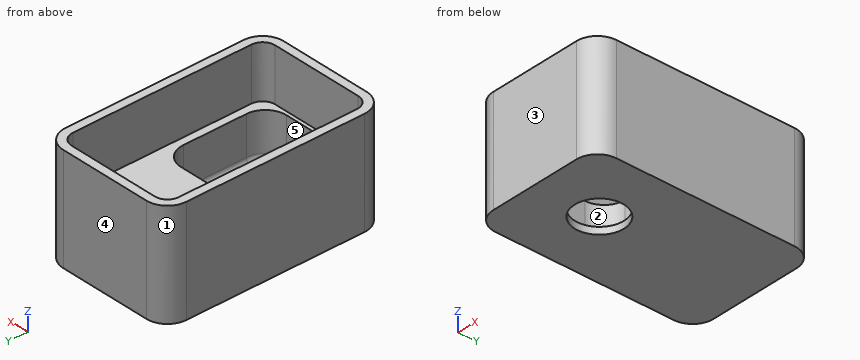
from build123d import *

# Parameters (mm, degrees)
SKETCH1_W           = 38.3
SKETCH1_H           = 62.8
SKETCH1_W_2         = 33.5
SKETCH1_H_2         = 58
SKETCH1_W_3         = 29
SKETCH1_H_3         = 30
SKETCH1_R           = 7
BOSS_EXTRUDE1_DEPTH = 2
BOSS_EXTRUDE2_START = 2
SKETCH1_3_W         = 38.3
SKETCH1_3_H         = 62.8
SKETCH1_3_W_2       = 33.5
SKETCH1_3_H_2       = 58
SKETCH1_3_W_3       = 29
SKETCH1_3_H_3       = 30
BOSS_EXTRUDE2_DEPTH = 13
BOSS_EXTRUDE3_START = 15
SKETCH1_4_W         = 38.3
SKETCH1_4_H         = 62.8
SKETCH1_4_W_2       = 33.5
SKETCH1_4_H_2       = 58
BOSS_EXTRUDE3_DEPTH = 15
FILLET1_R           = 3.6
FILLET2_R           = 6
FILLET3_R           = 2


with BuildPart() as part:
    # Sketch1 → Boss-Extrude1 (new body)
    # profile 1 of 3: a face of its own
    with BuildSketch(Plane.XY):
        with Locations((0, 13)):
            Rectangle(SKETCH1_W, SKETCH1_H)
        with Locations((0, 13)):
            Rectangle(SKETCH1_W_2, SKETCH1_H_2, mode=Mode.SUBTRACT)
    # profile 2 of 3: a face of its own
    with BuildSketch(Plane.XY):
        with Locations((0, 13)):
            Rectangle(SKETCH1_W_2, SKETCH1_H_2)
        Rectangle(SKETCH1_W_3, SKETCH1_H_3, mode=Mode.SUBTRACT)
    # profile 3 of 3: a face of its own
    with BuildSketch(Plane.XY):
        Rectangle(SKETCH1_W_3, SKETCH1_H_3)
        Circle(SKETCH1_R, mode=Mode.SUBTRACT)
    extrude(amount=BOSS_EXTRUDE1_DEPTH)

    # Sketch1<3> → Boss-Extrude2 (add)
    # profile 1 of 2: a face of its own
    with BuildSketch(Plane.XY.offset(BOSS_EXTRUDE2_START)):
        with Locations((0, 13)):
            Rectangle(SKETCH1_3_W, SKETCH1_3_H)
        with Locations((0, 13)):
            Rectangle(SKETCH1_3_W_2, SKETCH1_3_H_2, mode=Mode.SUBTRACT)
    # profile 2 of 2: a face of its own
    with BuildSketch(Plane.XY.offset(BOSS_EXTRUDE2_START)):
        with Locations((0, 13)):
            Rectangle(SKETCH1_3_W_2, SKETCH1_3_H_2)
        Rectangle(SKETCH1_3_W_3, SKETCH1_3_H_3, mode=Mode.SUBTRACT)
    extrude(amount=BOSS_EXTRUDE2_DEPTH)

    # Sketch1<4> → Boss-Extrude3 (add)
    with BuildSketch(Plane.XY.offset(BOSS_EXTRUDE3_START)):
        with Locations((0, 13)):
            Rectangle(SKETCH1_4_W, SKETCH1_4_H)
        with Locations((0, 13)):
            Rectangle(SKETCH1_4_W_2, SKETCH1_4_H_2, mode=Mode.SUBTRACT)
    extrude(amount=BOSS_EXTRUDE3_DEPTH)

    # Fillet1
    fillet1_edges = [part.edges().sort_by_distance(p)[0] for p in [
        (-16.75, 42, 22.5),
        (-16.75, -16, 22.5),
        (16.75, -16, 22.5),
        (16.75, 42, 22.5),
    ]]
    fillet(fillet1_edges, radius=FILLET1_R)

    # Fillet2
    fillet2_edges = [part.edges().sort_by_distance(p)[0] for p in [
        (19.15, -18.4, 15),
        (-19.15, -18.4, 15),
        (-19.15, 44.4, 15),
        (19.15, 44.4, 15),
        (14.5, -15, 8.5),
        (14.5, 15, 8.5),
        (-14.5, 15, 8.5),
        (-14.5, -15, 8.5),
    ]]
    fillet(fillet2_edges, radius=FILLET2_R)

    # Fillet3
    fillet3_edges = [part.edges().sort_by_distance(p)[0] for p in [
        (-14.5, 0, 2),
        (0, -15, 2),
        (14.5, 0, 2),
        (0, 15, 2),
        (12.742640687, 13.242640687, 2),
        (12.742640687, -13.242640687, 2),
        (-12.742640687, 13.242640687, 2),
        (-12.742640687, -13.242640687, 2),
    ]]
    fillet(fillet3_edges, radius=FILLET3_R)


solid = part.part
Can you work these out from the model? Positions are in its coordinate system, mm. Face numbers are marked on the shaded views. A direction names the side the tool comes from. Give positions to 0.01 mm unless a question says otherwise; leave off trailing zeros. Loops run counter-clockwise (first coordinate to the right, second up) from the corner with the lowest first, then second, coordinate; pieces in that order, holes last. Notation, with made-up numbers: (48.25, 88.25) - (68.25, 88.25) arc R28 cw to (68.25, 119.25) - close; hole circle Ø8 at (52.25, -20.5). An arc over 180 degrees is marked (long way). One line per item, written item: value.
(1) If we section it at C-C, the plane z = 8.5: List the corners of the cut face in (x, y) for me.
Verdict:
outline: (-19.15, -12.4) arc R6 ccw to (-13.15, -18.4) - (13.15, -18.4) arc R6 ccw to (19.15, -12.4) - (19.15, 38.4) arc R6 ccw to (13.15, 44.4) - (-13.15, 44.4) arc R6 ccw to (-19.15, 38.4) - close; hole (-14.5, -9) arc R6 ccw to (-8.5, -15) - (8.5, -15) arc R6 ccw to (14.5, -9) - (14.5, 9) arc R6 ccw to (8.5, 15) - (-8.5, 15) arc R6 ccw to (-14.5, 9) - close
(2) If we section it at B-B, the plane x = 0: List the corners of the cut face in (y, z) for me.
Verdict:
outline: (-18.4, 0) - (-7, 0) - (-7, 2) - (-13, 2) arc R2 cw to (-15, 4) - (-15, 15) - (-16, 15) - (-16, 30) - (-18.4, 30) - close; (7, 0) - (44.4, 0) - (44.4, 30) - (42, 30) - (42, 15) - (15, 15) - (15, 4) arc R2 cw to (13, 2) - (7, 2) - close
(3) If we section it at A-A, the plane y = 0: List the corners of the cut face in (x, z) for me, plus the area to 3 significant figures.
Verdict:
outline: (-19.15, 0) - (-7, 0) - (-7, 2) - (-12.5, 2) arc R2 cw to (-14.5, 4) - (-14.5, 15) - (-16.75, 15) - (-16.75, 30) - (-19.15, 30) - close; (7, 0) - (19.15, 0) - (19.15, 30) - (16.75, 30) - (16.75, 15) - (14.5, 15) - (14.5, 4) arc R2 cw to (12.5, 2) - (7, 2) - close
area: 243 mm^2
(4) I need wall thicknesses on line 1 along X through (y, z) = (-10, 27.75); line 2 along X through (y, z) = (8, 11.75); line 3 along Y through (x, z) = (0, 1.05). Which ranges of each line are inside material? Lowest first, please.
Verdict:
line 1: -19.15 to -16.75, 16.75 to 19.15
line 2: -19.15 to -14.5, 14.5 to 19.15
line 3: -18.4 to -7, 7 to 44.4
(5) I'm going to push flat-ended pins straight in: pin 1 (1 mm diameter, centred on x = 4, y = -3.5, fed in from +Z); pin 2 (3 mm diameter, centred on x = 8.5, y = 12, fed in from -Z); pin 3 (12.5 mm diameter, centred on x = -2, y = 5.5, fed in from +Z). Where does each tip first touch, or does it pass through?
Verdict:
pin 1: through
pin 2: z = 0
pin 3: z = 2
(6) If we section it at D-D, the plane y = 29: List the corners of the cut face in (x, z) for me.
Verdict:
outline: (-19.15, 0) - (19.15, 0) - (19.15, 30) - (16.75, 30) - (16.75, 15) - (-16.75, 15) - (-16.75, 30) - (-19.15, 30) - close
(7) If we mould it in two halves opening along X, with no side actions, what happens to the marked faces 1, 2 and 3? For each: released by +X, released by -X, zero draft, split by the parting line, or undercut.
Verdict:
face 1: released by -X
face 2: undercut
face 3: zero draft
(8) On a 3-axis mill with a long thin cutter (end or side, diameter ignored), from which of +Z, -Z, +X, -X, +Y, -Y can I reach the whole of each face in a straight line? I mean the marked faces 4 and 5. Say none if no direction works.
Verdict:
face 4: +Z, -Z, +X, -X, +Y
face 5: +Z
